from build123d import *

# Parameters (mm, degrees)
ESBO_O1_W                                            = 18
ESBO_O1_H                                            = 500
RESSALTO_EXTRUS_O1_DEPTH                             = 7
FURO_DE_DI_METRO_2_0_2_1_D                           = 2
FURO_DE_DI_METRO_6_0_6_1_D                           = 6
REBAIXO_PARA_PARAFUSO_DE_M_QUINA_DE_CABE_D           = 3.5
REBAIXO_PARA_PARAFUSO_DE_M_QUINA_DE_CABE_CBORE_D     = 6
REBAIXO_PARA_PARAFUSO_DE_M_QUINA_DE_CABE_CBORE_DEPTH = 3.5
PADR_O_LINEAR1_COUNT                                 = 16
PADR_O_LINEAR1_PITCH                                 = 30
PADR_O_LINEAR2_COUNT                                 = 17
PADR_O_LINEAR2_PITCH                                 = 30
CHANFRO1_SIZE                                        = 0.3


with BuildPart() as part:
    # Esboço1 → Ressalto-extrusão1 (new body)
    with BuildSketch(Plane.XZ):
        with Locations((-9, -250)):
            Rectangle(ESBO_O1_W, ESBO_O1_H)
    extrude(amount=-RESSALTO_EXTRUS_O1_DEPTH)

    # Furo de diâmetro Ø2.0 (2)1 (through all)
    with Locations(Plane(origin=(0, 0, -500), x_dir=(-1, 0, 0), z_dir=(0, 0, -1))):
        with Locations((0, 4.7), (18, 4.7)):
            Hole(FURO_DE_DI_METRO_2_0_2_1_D / 2)

    # Furo de diâmetro Ø6.0 (6)1 (through all)
    with Locations(Plane(origin=(0, 7, 0), x_dir=(1, 0, 0), z_dir=(0, 1, 0))):
        with Locations((-9, 25)):
            furo_de_di_metro_6_0_6_1 = Hole(FURO_DE_DI_METRO_6_0_6_1_D / 2)

    # Rebaixo para parafuso de máquina de cabeça sextavada de M31 (through all)
    with Locations(Plane(origin=(0, 7, 0), x_dir=(1, 0, 0), z_dir=(0, 1, 0))):
        with Locations((-9, 10)):
            rebaixo_para_parafuso_de_m_quina_de_cabe = CounterBoreHole(REBAIXO_PARA_PARAFUSO_DE_M_QUINA_DE_CABE_D / 2, REBAIXO_PARA_PARAFUSO_DE_M_QUINA_DE_CABE_CBORE_D / 2, REBAIXO_PARA_PARAFUSO_DE_M_QUINA_DE_CABE_CBORE_DEPTH)

    # Padrão linear1: Furo de diâmetro Ø6.0 (6)1 ×16
    with Locations(*[(0, 0, -i * PADR_O_LINEAR1_PITCH) for i in range(1, PADR_O_LINEAR1_COUNT)]):
        add(furo_de_di_metro_6_0_6_1, mode=Mode.SUBTRACT)

    # Padrão linear2: Rebaixo para parafuso de máquina de cabeça sextavada de M31 ×17
    with Locations(*[(0, 0, -i * PADR_O_LINEAR2_PITCH) for i in range(1, PADR_O_LINEAR2_COUNT)]):
        add(rebaixo_para_parafuso_de_m_quina_de_cabe, mode=Mode.SUBTRACT)

    # Chanfro1
    chanfro1_edges = [part.edges().sort_by_distance(p)[0] for p in [
        (0, 7, -250),
        (-18, 7, -250),
        (0, 0, -250),
        (-18, 0, -250),
    ]]
    chamfer(chanfro1_edges, length=CHANFRO1_SIZE)


solid = part.part
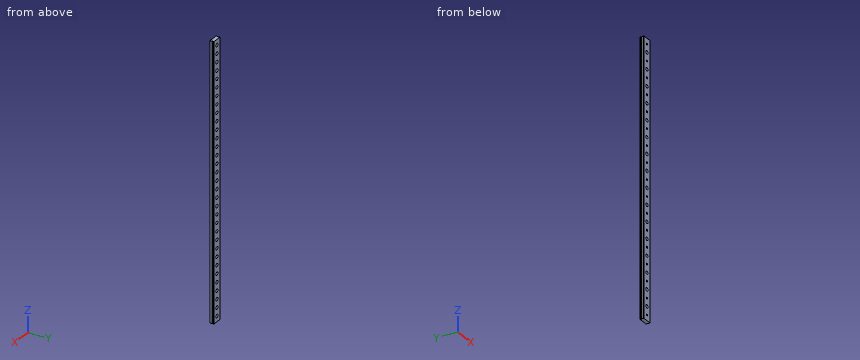
Verification items for the finished model (mm, model axes). Round coordinates to 2 decimals unless told otherwise and drop trailing zeros. Answer in a Markdown table with one row per item. Add a question column.
Q1. Material ranges on line 1 (X direction, y = 2.5, z = -445); line 2 (X direction, y = 1.4, z = -160), recorded low to high.
Q2. Section check A-A on y = 1.5. State how many separate pieces and enclosed holes the cut face has, plus the area to 3 significant figures.
Q3. Gauge pin test, flat end, axial feed: pin 1 (4.5 mm diameter, centred on x = -9, z = -400, fed in from +Y). Record the tip position at first contact, or that the pin passes through.
Found:
| question | item | result |
|---|---|---|
| 1 | line 1 | x = -18 to -12, -6 to 0 |
| 1 | line 2 | x = -18 to -10.75, -7.25 to 0 |
| 2 | separate pieces | 1 |
| 2 | enclosed holes | 33 |
| 2 | area | 8,380 mm² |
| 3 | pin 1 | stops at y = 3.5 |
